Verification items for this drawing (mm, ordinates from the low corner). A direction names the side the tool comes from. Coordinates: 2 decimals unless noted, no trailing zeros. Loops run counter-clockwise (first coordinate to the right, second up) from the corner with the lowest first, then second, coordinate; pieces in that order, holes last. Notation, with made-up numbers: M 20,83.25 L 39,83.25 A3 ccw 39,88.25 Z; hole C -19,40 d9. An arc over 180 degrees is marked long. Use CSV: the item, a comma, the result in double quotes.
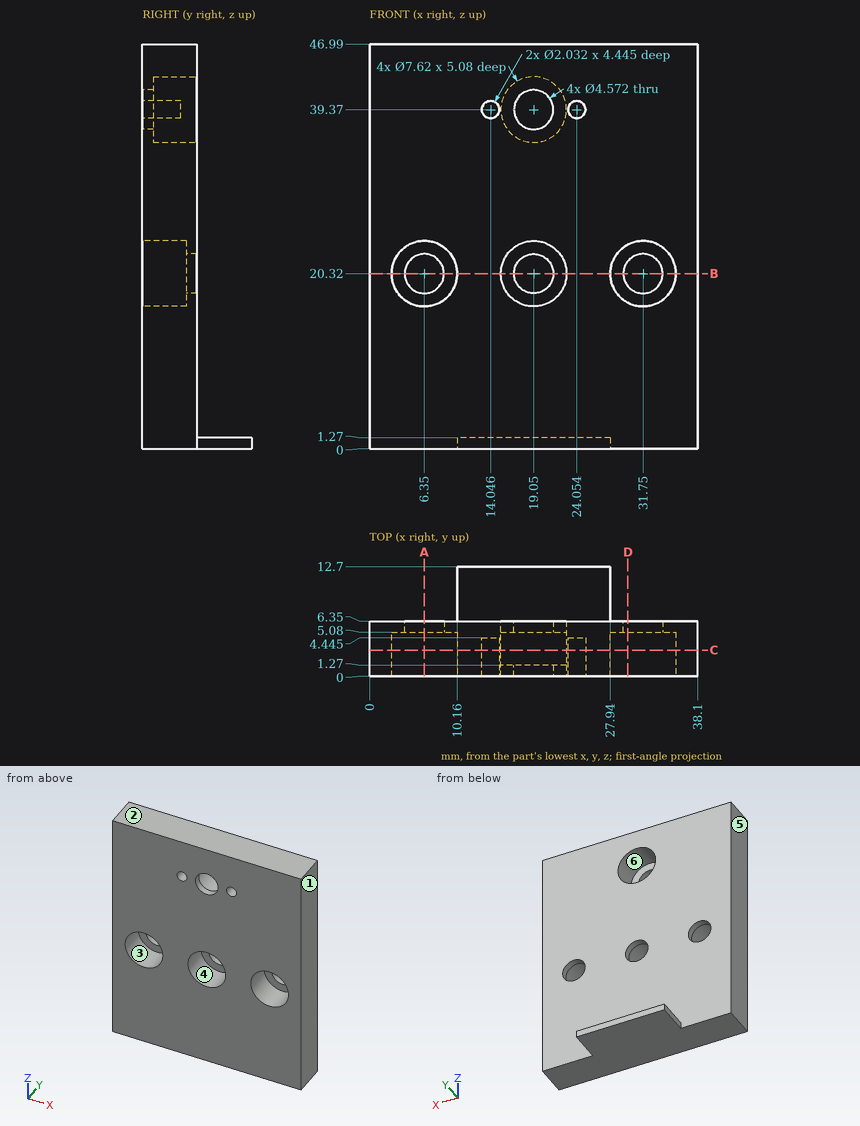
1. Section check B-B, the plane z = 20.32. Record the cut outline in (x, y), plus the area to 3 significant figures.
The answers:
outline,"M 0,0 L 2.54,0 L 2.54,5.08 L 4.06,5.08 L 4.06,6.35 L 0,6.35 Z; M 8.64,5.08 L 10.16,5.08 L 10.16,0 L 15.24,0 L 15.24,5.08 L 16.76,5.08 L 16.76,6.35 L 8.64,6.35 Z; M 21.34,5.08 L 22.86,5.08 L 22.86,0 L 27.94,0 L 27.94,5.08 L 29.46,5.08 L 29.46,6.35 L 21.34,6.35 Z; M 34.04,5.08 L 35.56,5.08 L 35.56,0 L 38.1,0 L 38.1,6.35 L 34.04,6.35 Z"
area,"108 mm^2"
2. Gauge pin test, flat ends, axial feed: P1, Ø3, axis at x = 22.5, z = 35, coming from the +Y side; P2, Ø1.4, axis at y = 10, z = 0.5, coming from the +X side; P3, Ø4, axis at x = 5, z = 20.5, coming from the -Y side; P4, Ø4.5, axis at x = 19.05, z = 20.32, coming from the -Y side. Record the tip position at first contact, or that the pin passes through.
The answers:
P1,"y = 6.35"
P2,"x = 27.94"
P3,"y = 5.08"
P4,"through"
3. Thickness scan on line 1 (Z direction, x = 19.05, y = 1.4); line 2 (Z direction, x = 31.75, y = 4.05); line 3 (Z direction, x = 6.35, y = 5.9). Record the ranges inside material, lowest first. Write a range as [from, to].
The answers:
line 1,"[0, 16.51], [24.13, 35.56], [43.18, 46.99]"
line 2,"[0, 16.51], [24.13, 46.99]"
line 3,"[0, 18.03], [22.61, 46.99]"
4. Section check C-C, the plane y = 3. Record the cut outline in (x, z).
The answers:
outline,"M 0,0 L 38.1,0 L 38.1,46.99 L 0,46.99 Z; hole C 6.35,20.32 d7.62; hole C 14.05,39.37 d2.03; hole C 19.05,20.32 d7.62; hole C 19.05,39.37 d7.62; hole C 24.05,39.37 d2.03; hole C 31.75,20.32 d7.62"
5. Section check D-D, the plane x = 30. Record the cut outline in (y, z), plus the area to 3 significant figures.
The answers:
outline,"M 0,0 L 6.35,0 L 6.35,18.85 L 5.08,18.85 L 5.08,16.94 L 0,16.94 Z; M 0,23.7 L 5.08,23.7 L 5.08,21.79 L 6.35,21.79 L 6.35,46.99 L 0,46.99 Z"
area,"260 mm^2"
6. Release check for a two-part mould opening along Z. For the marked faces 1, 2 and 3 record: +Z half, -Z half, draft (parallel to the pull), parting line (faces both ways), or undercut.
The answers:
face 1,"draft"
face 2,"+Z half"
face 3,"undercut"
7. Set-up check for the marked faces 4, 5 and 6: record each of +Z, -Z, +X, -X, +Y, -Y from which the full face is reachable in a straight line by a thin tool's end or side.
The answers:
face 4,"-Y"
face 5,"+Z, -Z, -X, +Y, -Y"
face 6,"+Y"
8. Section check A-A, the plane x = 6.35. Record the cut outline in (y, z), plus the area to 3 significant figures.
The answers:
outline,"M 0,0 L 6.35,0 L 6.35,18.03 L 5.08,18.03 L 5.08,16.51 L 0,16.51 Z; M 0,24.13 L 5.08,24.13 L 5.08,22.61 L 6.35,22.61 L 6.35,46.99 L 0,46.99 Z"
area,"254 mm^2"
